Source: CAD feature listing. Evaluate the final solid. Frame: model axes, mm. A direction names the side the tool comes from. Round coordinates to 2 decimals unless told otherwise and drop trailing zeros. Loops run counter-clockwise (first coordinate to the right, second up) from the corner with the lowest first, then second, coordinate; pieces in that order, holes last. Notation, with made-up numbers: M 17,53.5 L 70,53.5 A17 ccw 70,67.5 Z; hole C -36,-30 d11. An arc over 180 degrees is marked long. Answer as a JSON object with one key per item and string values.
from build123d import *

# Parameters (mm, degrees)
SKETCH1_R                = 8
SKETCH1_R_2              = 6.75
BOSS_EXTRUDE1_DEPTH      = 1000
BOSS_EXTRUDE1_2_DEPTH    = 1000
BOSS_EXTRUDE2_DEPTH      = 75
BOSS_EXTRUDE2_DEPTH_BACK = 75
SKETCH2_R                = 8
SKETCH2_R_2              = 6.75
CUT_EXTRUDE1_START       = -150
SKETCH3_R                = 6.75
CUT_EXTRUDE1_DEPTH       = 150
BOSS_EXTRUDE3_DEPTH      = 75
BOSS_EXTRUDE3_DEPTH_BACK = 75
SKETCH4_R                = 8
SKETCH4_R_2              = 6.75
SKETCH6_R                = 6.75
CUT_EXTRUDE2_DEPTH       = 150


with BuildPart() as part:
    # Sketch1 → Boss-Extrude1 (new body)
    with BuildSketch(Plane(origin=(0, 0, 0), x_dir=(0, 0, -1), z_dir=(1, 0, 0))):
        with Locations((-50, 0)):
            Circle(SKETCH1_R)
        with Locations((-50, 0)):
            Circle(SKETCH1_R_2, mode=Mode.SUBTRACT)
    extrude(amount=BOSS_EXTRUDE1_DEPTH)



with BuildPart() as body_2:
    # Sketch1 → Boss-Extrude1 2 (new body)
    with BuildSketch(Plane(origin=(0, 0, 0), x_dir=(0, 0, -1), z_dir=(1, 0, 0))):
        with Locations((50, 0)):
            Circle(SKETCH1_R)
        with Locations((50, 0)):
            Circle(SKETCH1_R_2, mode=Mode.SUBTRACT)
    extrude(amount=BOSS_EXTRUDE1_2_DEPTH)


with BuildPart() as part_1:
    add(part.part)

    add(body_2.part)  # Boss-Extrude2 merges body 2
    # Sketch2 → Boss-Extrude2 (add, two sides: drawn at the far end of the back side and taken through both)
    with BuildSketch(Plane.XY.offset(-BOSS_EXTRUDE2_DEPTH_BACK)):
        Circle(SKETCH2_R)
        Circle(SKETCH2_R_2, mode=Mode.SUBTRACT)
    extrude(amount=BOSS_EXTRUDE2_DEPTH + BOSS_EXTRUDE2_DEPTH_BACK)

    # Sketch3 → Cut-Extrude1 (cut)
    with BuildSketch(Plane.XY.offset(75).offset(CUT_EXTRUDE1_START)):
        Circle(SKETCH3_R)
    extrude(amount=CUT_EXTRUDE1_DEPTH, mode=Mode.SUBTRACT)

    # Sketch4 → Boss-Extrude3 (add, two sides: drawn at the far end of the back side and taken through both)
    with BuildSketch(Plane.XY.offset(-BOSS_EXTRUDE3_DEPTH_BACK)):
        with Locations((1000, 0)):
            Circle(SKETCH4_R)
        with Locations((1000, 0)):
            Circle(SKETCH4_R_2, mode=Mode.SUBTRACT)
    extrude(amount=BOSS_EXTRUDE3_DEPTH + BOSS_EXTRUDE3_DEPTH_BACK)

    # Sketch6 → Cut-Extrude2 (cut)
    with BuildSketch(Plane.XY.offset(75)):
        with Locations((1000, 0)):
            Circle(SKETCH6_R)
    extrude(amount=-CUT_EXTRUDE2_DEPTH, mode=Mode.SUBTRACT)


solid = part_1.part
Item 1: Section A-A on y = 0. Give the number of separate pieces and of enclosed holes in the cut face, then the cut area to 3 significant figures.
Answer sheet:
{"separate pieces": "3", "enclosed holes": "3", "area": "5,670 mm²"}
Item 2: Contact query for flat-ended pins moving along their axis: pin 1 Ø1.5 at (x, y) = (708.5, -4) entering from +Z; pin 2 Ø1 at (x, y) = (395.5, -3.5) entering from +Z; pin 3 Ø1.5 at (x, y) = (900.5, -5.5) entering from +Z. Output: stop coordinate, or through.
Answer sheet:
{"pin 1": "stops at z = 57.31", "pin 2": "stops at z = 57.42", "pin 3": "stops at z = 56.44"}
Item 3: Section C-C on z = -6. Return the cut outline in (x, y).
Answer sheet:
{"outline": "C 0,0 d16; C 1000,0 d16; hole C 0,0 d13.5; hole C 1000,0 d13.5"}
Item 4: Access query for faces 1 (the flat face through (996, -6, -75)), 2 (the cylindrical face through (493, -4.868, -43.651)). Directions: +Z, -Z, +X, -X, +Y, -Y. A direction counts if a zero-diameter tool reaches every point of the face in a straight line with its end or side. Return the directions, or none.
Answer sheet:
{"face 1": "-Z, +X, -X, +Y, -Y", "face 2": "none"}
Item 5: Section B-B on x = 607. Return the cut outline in (y, z), then the cut area to 3 significant figures.
Answer sheet:
{"outline": "C 0,-50 d16; C 0,50 d16; hole C 0,-50 d13.5; hole C 0,50 d13.5", "area": "116 mm²"}
Item 6: Line query: probe 1 along Z at (x, y) = (622.5, 0); probe 2 along Y at (x, z) = (0, 21.5); probe 3 along Z at (x, y) = (758.5, -4.25). Output: solid intervals per line, ascending. Write a range as from..to.
Answer sheet:
{"probe 1": "z = -58..-56.75, -43.25..-42, 42..43.25, 56.75..58", "probe 2": "y = -8..-6.75, 6.75..8", "probe 3": "z = -56.78..-55.24, -44.76..-43.22, 43.22..44.76, 55.24..56.78"}
